Input: dimensioned drawing with shaded views. Units: mm. Origin: part minimum x, y, z. A direction names the side the tool comes from. Round coordinates to 2 decimals unless told otherwise and drop trailing zeros. Loops run counter-clockwise (first coordinate to the right, second up) from the corner with the lowest first, then second, coordinate; pieces in that order, holes last. Notation, with made-up numbers: M 11.5,-5.5 L 56.5,-5.5 A16 ccw 56.5,13.5 Z; hole C -16,65 d10. An arc over 180 degrees is marked long. Use one line per item in the form item = value. Start each with the question number.
Q1. First-contact query: P1, Ø1.4, axis at x = 7, z = 8.5, coming from the +Y side. Flat tip, straight axial feed; report the tip coordinate or a pass-through.
Q2. Ray query, line 1 along Z through (x, y) = (8, 8) (3 decimals); line 2 along Z through (x, y) = (12, 7). Return the intervals inside material, ascending.
Q3. Mould query, pull axis X, two halves, no side actions, for the marked faces 1, 2 and 3. Classes: pulls with the +X half, pulls with the -X half, needs draft (parallel to the pull), parting line crosses it, or undercut.
Q4. Section query A-A, the plane y = 10. Output: boundary loops of the cut face in (x, z) (3 decimals), and give its area (3 significant figures).
Q5. Section query B-B, the plane z = 12. Output: boundary loops of the cut face in (x, y).
Q6. Section query C-C, the plane x = 4. Output: boundary loops of the cut face in (y, z).
Q7. Access query for the marked faces 4, 5 and 6. Directions: +Z, -Z, +X, -X, +Y, -Y. A direction counts if a zero-diameter tool reaches every point of the face in a straight line with its end or side. Return the directions, or none.
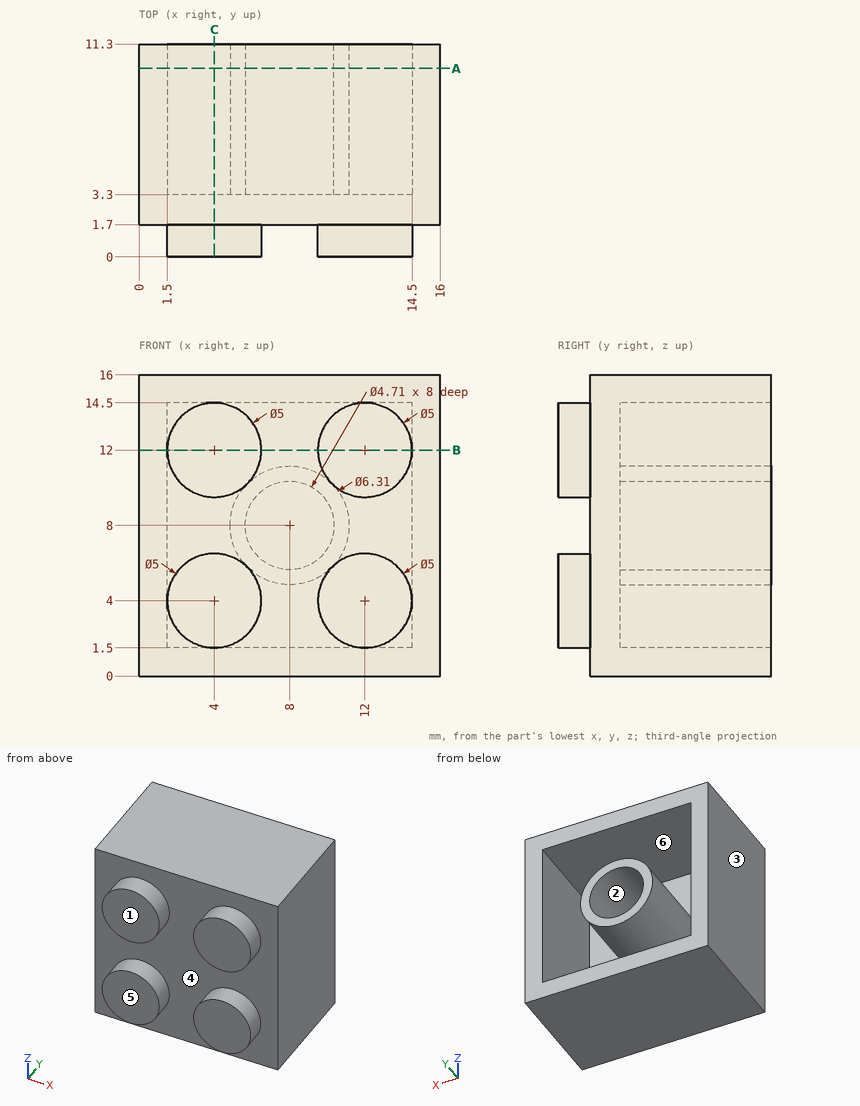
Results found:
q1.P1 = 3.3
q2.line_1 = 0 to 1.5, 4.845 to 5.645, 10.355 to 11.155, 14.5 to 16
q2.line_2 = 0 to 1.5, 14.5 to 16
q3.face_1 = needs draft
q3.face_2 = undercut
q3.face_3 = pulls with the -X half
q4.outline = M 0,0 L 16,0 L 16,16 L 0,16 Z; C 8,8 d6.31; hole M 1.5,1.5 L 14.5,1.5 L 14.5,14.5 L 1.5,14.5 Z; hole C 8,8 d4.71
q4.area = 101 mm²
q5.outline = M 0,1.7 L 1.5,1.7 L 1.5,0 L 6.5,0 L 6.5,1.7 L 9.5,1.7 L 9.5,0 L 14.5,0 L 14.5,1.7 L 16,1.7 L 16,11.3 L 14.5,11.3 L 14.5,3.3 L 1.5,3.3 L 1.5,11.3 L 0,11.3 Z
q6.outline = M 0,1.5 L 1.7,1.5 L 1.7,0 L 11.3,0 L 11.3,1.5 L 3.3,1.5 L 3.3,14.5 L 11.3,14.5 L 11.3,16 L 1.7,16 L 1.7,14.5 L 0,14.5 L 0,9.5 L 1.7,9.5 L 1.7,6.5 L 0,6.5 Z
q7.face_4 = -Y
q7.face_5 = +Z, -Z, +X, -X, -Y
q7.face_6 = +Y
